The listing builds one solid part. Answer for the finished solid, in the listing's coordinates (mm). A direction names the side the tool comes from. Coordinates: 2 decimals unless noted, no trailing zeros. Loops run counter-clockwise (first coordinate to the right, second up) from the corner with the lowest first, then second, coordinate; pieces in that order, holes last. Notation, with made-up numbers: (28.25, 33) -> (53.25, 33) arc R10 ccw to (53.25, 44) -> close; hole circle Ø4 at (86, 65). An arc over 180 degrees is marked (long way). Answer in a Markdown table with one row per item.
Autodesk Inventor part; units mm, degrees
ref_plane "YZ Plane" through (0, 0, 0) normal (1, 0, 0) x (0, 1, 0)
ref_plane "XZ Plane" through (0, 0, 0) normal (0, 1, 0) x (-1, 0, 0)
ref_plane "XY Plane" through (0, 0, 0) normal (0, 0, 1) x (1, 0, 0)
sketch "Sketch1" plane through (0, 0, 0) normal (1, 0, 0) x (0, 1, 0)
  line L0 (0, 0) -> (50.8, 0)
  line L1 (50.8, 0) -> (50.8, -101.6)
  line L2 (50.8, -101.6) -> (0, -101.6)
  line L3 (0, -101.6) -> (0, 0)
  dimension "d0" = 50.8
  dimension "d1" = 101.6
extrude "Extrusion1" add sketch "Sketch1" along normal blind 254
sketch "Sketch2" plane through (0, 0, 0) normal (0, 0, 1) x (1, 0, 0)
  line L0 (0, 0) -> (0, 50.8)
  line L1 (0, 0) -> (254, 0)
  line L2 (254, 50.8) -> (254, 0)
  line L3 (0, 50.8) -> (254, 50.8)
  line L4 (0, 0) -> (254, 0)
  line L5 (50.8, 0) -> (50.8, 3.81)
  line L6 (50.8, 3.81) -> (0, 3.81)
  line L7 (0, 0) -> (0, 50.8)
  line L8 (127, 0) -> (127, 50.8) construction
  line L9 (203.2, 0) -> (203.2, 3.81)
  line L10 (203.2, 3.81) -> (254, 3.81)
  line L11 (50.8, 0) -> (0, 0)
  line L12 (203.2, 0) -> (254, 0)
  line L13 (254, 50.8) -> (254, 0)
  line L14 (254, 3.81) -> (254, 0)
  dimension "d4" = 3.81
  dimension "d5" = 90
  dimension "d6" = 50.8
extrude "Extrusion2" cut sketch "Sketch2" against normal up to next contours L0 L6 L5 L1 | L9 L10 L2 L1
properties part number "lifterBase"
Item 1: Find the intervals of material crossed by probe 1 along Y at (x, z) = (18, -73), in increasing order.
Findings below:
| item | result |
|---|---|
| probe 1 | y = 3.81 to 50.8 |
Item 2: Determine the mould class of faces 1 (the face through (126, 0, -52)), 2 (the face through (125, 50.8, -50)), 3 (the face through (254, 27, -50)) for opening direction Y: +Y half, -Y half, draft (parallel to the pull), parting line (faces both ways), or undercut.
Findings below:
| item | result |
|---|---|
| face 1 | -Y half |
| face 2 | +Y half |
| face 3 | draft |
Item 3: A cutting plane is placed at B-B, the plane x = 35.5. Determine the outline of the cut face in (y, z), plus the area to 3 significant figures.
Findings below:
| item | result |
|---|---|
| outline | (3.81, -101.6) -> (50.8, -101.6) -> (50.8, 0) -> (3.81, 0) -> close |
| area | 4,770 mm2 |
Item 4: A tool of negligible diameter and unlimited length cuts with its end or side. For faces 4 (the face through (26, 3.81, -50)), 5 (the face through (0, 27, -50)), 6 (the face through (228, 3.81, -50)), from which of +Z, -Z, +X, -X, +Y, -Y can it reach the whole face along a straight path? Write none if from no direction.
Findings below:
| item | result |
|---|---|
| face 4 | +Z, -Z, -X, -Y |
| face 5 | +Z, -Z, -X, +Y, -Y |
| face 6 | +Z, -Z, +X, -Y |
Item 5: A cutting plane is placed at A-A, the plane z = -24. Determine the outline of the cut face in (x, y).
Findings below:
| item | result |
|---|---|
| outline | (0, 3.81) -> (50.8, 3.81) -> (50.8, 0) -> (203.2, 0) -> (203.2, 3.81) -> (254, 3.81) -> (254, 50.8) -> (0, 50.8) -> close |
Item 6: Flat-ended cylindrical pins translate along their axes: pin 1 Ø5 at (x, z) = (211, -44) entering from -Y; pin 2 Ø1.9 at (y, z) = (1.5, -48) entering from -X; pin 3 Ø4 at (y, z) = (1, -72) entering from +X. Find the tip coordinate at first contact, or state that the pin passes through.
Findings below:
| item | result |
|---|---|
| pin 1 | stops at y = 3.81 |
| pin 2 | stops at x = 50.8 |
| pin 3 | stops at x = 203.2 |
